```python
from build123d import *

# Parameters (mm, degrees)
SALIENTE_EXTRUIR1_DEPTH = 60
CROQUIS4_W              = 60
CROQUIS4_H              = 6
SALIENTE_EXTRUIR3_DEPTH = 1
CROQUIS5_R              = 2.75
CORTAR_EXTRUIR1_DEPTH   = 25
CROQUIS6_R              = 6
CORTAR_EXTRUIR2_DEPTH   = 8
REDONDEO1_R             = 10


with BuildPart() as part:
    # Croquis1 → Saliente-Extruir1 (new body)
    with BuildSketch(Plane.XY):
        Polygon((24, -100), (24, -20.5), (14, -20.5), (14, 0), (0, 0), (0, -100), align=None)
    extrude(amount=SALIENTE_EXTRUIR1_DEPTH)

    # Croquis4 → Saliente-Extruir3 (add)
    with BuildSketch(Plane(origin=(14, 0, 0), x_dir=(0, 0, -1), z_dir=(1, 0, 0))):
        with Locations((-30, -10)):
            Rectangle(CROQUIS4_W, CROQUIS4_H)
    extrude(amount=SALIENTE_EXTRUIR3_DEPTH)

    # Croquis5 → Cortar-Extruir1 (cut, through all)
    with BuildSketch(Plane.ZY):
        with Locations((15, -10)):
            Circle(CROQUIS5_R)
        with Locations((45, -10)):
            Circle(CROQUIS5_R)
    extrude(amount=-CORTAR_EXTRUIR1_DEPTH, mode=Mode.SUBTRACT)

    # Croquis6 → Cortar-Extruir2 (cut)
    with BuildSketch(Plane.ZY):
        with Locations((15, -10)):
            Circle(CROQUIS6_R)
        with Locations((45, -10)):
            Circle(CROQUIS6_R)
    extrude(amount=-CORTAR_EXTRUIR2_DEPTH, mode=Mode.SUBTRACT)

    # Redondeo1
    redondeo1_edges = [part.edges().sort_by_distance(p)[0] for p in [
        (24, -60.25, 0),
        (24, -60.25, 60),
    ]]
    fillet(redondeo1_edges, radius=REDONDEO1_R)


solid = part.part
```
Here's how the part is built. I have some questions about the finished solid (model axes, mm). A direction names the side the tool comes from. Coordinates: 2 decimals unless noted, no trailing zeros. Loops run counter-clockwise (first coordinate to the right, second up) from the corner with the lowest first, then second, coordinate; pieces in that order, holes last. Notation, with made-up numbers: M 64.5,27 L 93.5,27 A17 cw 93.5,31 Z; hole C 41.5,-39 d10. An arc over 180 degrees is marked long. One line per item, written item: value.
1. Please list where these lines run through material, in increasing order: probe 1 along Z at (x, y) = (12, -7.5); probe 2 along Y at (x, z) = (5.25, 45); probe 3 along Y at (x, z) = (14.5, 52.5).
Geometry says:
probe 1: z = 0 to 13.85, 16.15 to 43.85, 46.15 to 60
probe 2: y = -100 to -16, -4 to 0
probe 3: y = -100 to -20.5, -13 to -7
2. Imagine slicing it at D-D (x = 2.5). List the corners of the cut face in (y, z) for me.
Geometry says:
outline: M -100,0 L 0,0 L 0,60 L -100,60 Z; hole C -10,15 d12; hole C -10,45 d12
3. Imagine slicing it at C-C (z = 32.5). List the corners of the cut face in (x, y) for me, and give its area (3 significant figures).
Geometry says:
outline: M 0,-100 L 24,-100 L 24,-20.5 L 14,-20.5 L 14,-13 L 15,-13 L 15,-7 L 14,-7 L 14,0 L 0,0 Z
area: 2,200 mm2
4. Thinking about a two-plate mould opening in Y: for faces 1 (the flat face through (7, 0, 30)), 2 (the cylindrical face through (21.15, -59.69, 3.01)), 3 (the cylindrical face through (11.451, -9.879, 12.253)), which applies, +Y half, -Y half, draft (parallel to the pull), parting line (faces both ways), or undercut?
Geometry says:
face 1: +Y half
face 2: draft
face 3: undercut
5. On a 3-axis mill with a long thin cutter (end or side, diameter ignored), from which of +Z, -Z, +X, -X, +Y, -Y can I reach the whole of each face in a straight line? I mean faces 4 (the flat face through (14, -17, 30)), 5 (the flat face through (8, -11, 18)), 6 (the flat face through (24, -61, 30)), 7 (the flat face through (15, -10, 30)), 8 (the flat face through (0, -49, 30)). Say none if no direction works.
Geometry says:
face 4: +Z, -Z, +X
face 5: -X
face 6: +Z, -Z, +X, +Y, -Y
face 7: +Z, -Z, +X, +Y
face 8: +Z, -Z, -X, +Y, -Y
6. Imagine slicing it at B-B (z = 15). List the corners of the cut face in (x, y) for me.
Geometry says:
outline: M 0,-100 L 24,-100 L 24,-20.5 L 14,-20.5 L 14,-13 L 15,-13 L 15,-12.75 L 8,-12.75 L 8,-16 L 0,-16 Z; M 0,-4 L 8,-4 L 8,-7.25 L 15,-7.25 L 15,-7 L 14,-7 L 14,0 L 0,0 Z
7. Will these pins go through, and if not, where does the flat tip stop? pin 1 Ø19 at (y, z) = (-10, 15) entering from +X; pin 2 Ø2 at (y, z) = (-16, 20.5) entering from +X; pin 3 Ø6 at (x, y) = (3, -79) entering from -Z; pin 4 Ø9 at (y, z) = (-10, 15) entering from -X.
Geometry says:
pin 1: stops at x = 15
pin 2: stops at x = 14
pin 3: stops at z = 0
pin 4: stops at x = 8
8. Imagine slicing it at A-A (y = -10). List the corners of the cut face in (x, z) for me.
Geometry says:
outline: M 0,0 L 15,0 L 15,12.25 L 8,12.25 L 8,9 L 0,9 Z; M 0,21 L 8,21 L 8,17.75 L 15,17.75 L 15,42.25 L 8,42.25 L 8,39 L 0,39 Z; M 0,51 L 8,51 L 8,47.75 L 15,47.75 L 15,60 L 0,60 Z
